Source: CAD feature listing. Evaluate the final solid. Frame: model axes, mm. A direction names the side the tool comes from. Coordinates: 2 decimals unless noted, no trailing zeros. Write each loop counter-clockwise with the first axis right and the second up, starting at its lowest first coordinate (ties: lowest second). Pieces come first, ordered by that corner, then holes. Notation, with made-up numbers: M 78,-4.75 L 124,-4.75 A37 cw 124,31.25 Z; hole C -24,-24 d8. An arc over 180 degrees is marked long. Write item = value, one per line. Start each with the question number.
1. Access query for faces 1 (the face through (14.251, 1.688, -5.637)), 2 (the face through (19.9, 1.7, -25)), 3 (the face through (5, 3, -13)). Directions: +Z, -Z, +X, -X, +Y, -Y. A direction counts if a zero-diameter tool reaches every point of the face in a straight line with its end or side. Return the directions, or none.
2. Line query: line 1 along Z through (x, y) = (2, 16.25); line 2 along X through (y, z) = (5.75, -10.25); line 3 along Z through (x, y) = (14, 3). Output: solid intervals per line, ascending.
3. Section query D-D (y = 7). Output: boundary loops of the cut face in (x, z) (3 decimals), then the cut area to 3 significant figures.
4. Section query A-A (y = 13). Output: boundary loops of the cut face in (x, z), then the cut area to 3 significant figures.
5. Pin query (flat end, axial travel): pin 1 Ø5 at (x, z) = (27.5, -3) entering from +Y; pin 2 Ø1.1 at (x, z) = (37.5, -22.5) entering from +Y; pin 3 Ø5 at (x, z) = (27, -8.5) entering from +Y. Return the tip coordinate at first contact, or that it passes through.
6. Section query B-B (y = 9.5). Output: boundary loops of the cut face in (x, z), then the cut area to 3 significant figures.
7. Pull-direction query (X, two-part tool) for faces 4 (the face through (2.5, 0, -12.3)), 5 (the face through (40, 9, -12)), 6 (the face through (16.479, 1.246, -17.874)); classes: pulls with the +X half, pulls with the -X half, needs draft (parallel to the pull), parting line crosses it, or undercut.
8. Section query C-C (x = 6). Output: boundary loops of the cut face in (y, z), then the cut area to 3 significant figures.
```python
from build123d import *

# Parameters (mm, degrees)
CROQUIS1_W              = 40
CROQUIS1_H              = 25
SALIENTE_EXTRUIR1_DEPTH = 18
CROQUIS2_R              = 16
CORTAR_EXTRUIR1_DEPTH   = 26
CROQUIS3_R              = 1.5
CORTAR_EXTRUIR2_DEPTH   = 19
CORTAR_EXTRUIR3_DEPTH   = 10
SALIENTE_EXTRUIR2_DEPTH = 25
CROQUIS6_W              = 1
CROQUIS6_H              = 25
SALIENTE_EXTRUIR3_DEPTH = 10


with BuildPart() as part:
    # Croquis1 → Saliente-Extruir1 (new body)
    with BuildSketch(Plane(origin=(0, 0, 0), x_dir=(1, 0, 0), z_dir=(0, 1, 0))):
        with Locations((20, 12.5)):
            Rectangle(CROQUIS1_W, CROQUIS1_H)
    extrude(amount=SALIENTE_EXTRUIR1_DEPTH)

    # Croquis2 → Cortar-Extruir1 (cut, through all)
    with BuildSketch(Plane.XY):
        with Locations((20, 18)):
            Circle(CROQUIS2_R)
    extrude(amount=-CORTAR_EXTRUIR1_DEPTH, mode=Mode.SUBTRACT)

    # Croquis3 → Cortar-Extruir2 (cut, through all)
    with BuildSketch(Plane(origin=(0, 18, 0), x_dir=(1, 0, 0), z_dir=(0, 1, 0))):
        with Locations((2, 2.5)):
            Circle(CROQUIS3_R)
        with Locations((2, 22.5)):
            Circle(CROQUIS3_R)
        with Locations((38, 2.5)):
            Circle(CROQUIS3_R)
        with Locations((38, 22.5)):
            Circle(CROQUIS3_R)
    extrude(amount=-CORTAR_EXTRUIR2_DEPTH, mode=Mode.SUBTRACT)

    # Croquis4 → Cortar-Extruir3 (cut)
    with BuildSketch(Plane.XZ):
        with BuildLine():
            Line((12.088237667, -6.478545635), (13.401635398, -5.142871626))
            Line((13.401635398, -5.142871626), (15.124961017, -6.145817155))
            ThreePointArc((15.124961017, -6.145817155), (15.475165724, -6.243431571), (15.828418521, -6.157499195))
            ThreePointArc((15.828418521, -6.157499195), (16.370055517, -5.897538787), (16.933440791, -5.688859407))
            ThreePointArc((16.933440791, -5.688859407), (17.240768872, -5.494639527), (17.414026723, -5.175024714))
            Line((17.414026723, -5.175024714), (17.890921137, -3.238966182))
            Line((17.890921137, -3.238966182), (19.764097728, -3.223214474))
            Line((19.764097728, -3.223214474), (20.273483375, -5.15097929))
            ThreePointArc((20.273483375, -5.15097929), (20.452091683, -5.467635229), (20.762642496, -5.656659312))
            ThreePointArc((20.762642496, -5.656659312), (21.329457457, -5.855834737), (21.875389609, -6.10664968))
            ThreePointArc((21.875389609, -6.10664968), (22.230037574, -6.186629256), (22.578551176, -6.083139256))
            Line((22.578551176, -6.083139256), (24.284766568, -5.051354413))
            Line((24.284766568, -5.051354413), (25.620440577, -6.364752144))
            Line((25.620440577, -6.364752144), (24.617495048, -8.088077763))
            ThreePointArc((24.617495048, -8.088077763), (24.519880632, -8.43828247), (24.605813007, -8.791535267))
            ThreePointArc((24.605813007, -8.791535267), (24.865773416, -9.333172263), (25.074452795, -9.896557537))
            ThreePointArc((25.074452795, -9.896557537), (25.268672676, -10.203885618), (25.588287488, -10.377143469))
            Line((25.588287488, -10.377143469), (27.524346021, -10.854037883))
            Line((27.524346021, -10.854037883), (27.540097728, -12.727214474))
            Line((27.540097728, -12.727214474), (25.612332912, -13.236600121))
            ThreePointArc((25.612332912, -13.236600121), (25.295676973, -13.415208429), (25.106652891, -13.725759242))
            ThreePointArc((25.106652891, -13.725759242), (24.907477465, -14.292574203), (24.656662522, -14.838506355))
            ThreePointArc((24.656662522, -14.838506355), (24.576682946, -15.19315432), (24.680172947, -15.541667922))
            Line((24.680172947, -15.541667922), (25.711957789, -17.247883314))
            Line((25.711957789, -17.247883314), (24.398560059, -18.583557323))
            Line((24.398560059, -18.583557323), (22.67523444, -17.580611794))
            ThreePointArc((22.67523444, -17.580611794), (22.325029732, -17.482997378), (21.971776936, -17.568929753))
            ThreePointArc((21.971776936, -17.568929753), (21.430139939, -17.828890162), (20.866754665, -18.037569541))
            ThreePointArc((20.866754665, -18.037569541), (20.6241928, -18.009408471), (20.386168733, -18.063941468))
            Line((20.386168733, -18.063941468), (19.909274319, -20))
            Line((19.909274319, -20), (18.036097728, -20.015751708))
            Line((18.036097728, -20.015751708), (17.526712081, -18.087986892))
            ThreePointArc((17.526712081, -18.087986892), (17.283728175, -18.036032676), (17.03755296, -18.069769637))
            ThreePointArc((17.03755296, -18.069769637), (16.470737999, -17.870594211), (15.924805848, -17.619779268))
            ThreePointArc((15.924805848, -17.619779268), (15.570157883, -17.539799692), (15.22164428, -17.643289693))
            Line((15.22164428, -17.643289693), (13.515428889, -18.675074535))
            Line((13.515428889, -18.675074535), (12.17975488, -17.361676805))
            Line((12.17975488, -17.361676805), (13.182700409, -15.638351186))
            ThreePointArc((13.182700409, -15.638351186), (13.280314825, -15.288146478), (13.194382449, -14.934893682))
            ThreePointArc((13.194382449, -14.934893682), (13.1083452, -14.769415199), (13.027105933, -14.601529171))
            ThreePointArc((13.027105933, -14.601529171), (13.02605148, -14.489666601), (13.109673231, -14.415358127))
            Line((13.109673231, -14.415358127), (16.284140051, -13.434659859))
            ThreePointArc((16.284140051, -13.434659859), (21.951688309, -11.884896122), (16.306733365, -10.25475669))
            Line((16.306733365, -10.25475669), (13.070699975, -9.410888594))
            ThreePointArc((13.070699975, -9.410888594), (12.983034926, -9.338706443), (12.981392618, -9.2251603))
            ThreePointArc((12.981392618, -9.2251603), (13.060028024, -9.055370844), (13.143532934, -8.887922594))
            ThreePointArc((13.143532934, -8.887922594), (13.22351251, -8.533274629), (13.12002251, -8.184761026))
            Line((13.12002251, -8.184761026), (12.088237667, -6.478545635))
        make_face()
        Polygon((5, -20), (5, -25), (0, -25), (0, -20), (0, -5), (0, 0), (5, 0), (5, -5), align=None)
        Polygon((35, 0), (35, -5), (35, -20), (35, -25), (40, -25), (40, -20), (40, -5), (40, 0), align=None)
    extrude(amount=-CORTAR_EXTRUIR3_DEPTH, mode=Mode.SUBTRACT)

    # Croquis5 → Saliente-Extruir2 (add)
    with BuildSketch(Plane(origin=(0, 0, -25), x_dir=(-1, 0, 0), z_dir=(0, 0, -1))):
        Polygon((-5, 10), (-5, 6), (-3.5, 10), align=None)
        Polygon((-35, 10), (-35, 6), (-36.5, 10), align=None)
    extrude(amount=-SALIENTE_EXTRUIR2_DEPTH)

    # Croquis6 → Saliente-Extruir3 (add)
    with BuildSketch(Plane.XZ.offset(-10)):
        with Locations((0.5, -12.5)):
            Rectangle(CROQUIS6_W, CROQUIS6_H)
        with Locations((39.5, -12.5)):
            Rectangle(CROQUIS6_W, CROQUIS6_H)
        with Locations((2.5, -12.5)):
            Rectangle(CROQUIS6_W, CROQUIS6_H)
        with Locations((37.5, -12.5)):
            Rectangle(CROQUIS6_W, CROQUIS6_H)
    extrude(amount=SALIENTE_EXTRUIR3_DEPTH)


solid = part.part
```
Results are:
q1.face_1 = +Y, -Y
q1.face_2 = -Z, +X, -X, +Y, -Y
q1.face_3 = +Z, -Z, -Y
q2.line_1 = -25 to -24, -21 to -4, -1 to 0
q2.line_2 = 0 to 1, 2 to 3, 5 to 9.71, 30.29 to 35, 37 to 38, 39 to 40
q2.line_3 = -25 to -18.38, -14.14 to -9.65, -5.49 to 0
q3.outline = M 0,-25 L 1,-25 L 1,0 L 0,0 Z; M 2,-25 L 3,-25 L 3,0 L 2,0 Z; M 4.625,-25 L 8.381,-25 L 8.381,0 L 4.625,0 Z; M 31.619,-25 L 35.375,-25 L 35.375,0 L 31.619,0 Z; M 37,-25 L 38,-25 L 38,0 L 37,0 Z; M 39,-25 L 40,-25 L 40,0 L 39,0 Z
q3.area = 288 mm^2
q4.outline = M 0,-25 L 4.8,-25 L 4.8,0 L 0,0 Z; M 35.2,-25 L 40,-25 L 40,0 L 35.2,0 Z; hole C 2,-22.5 d3; hole C 2,-2.5 d3; hole C 38,-22.5 d3; hole C 38,-2.5 d3
q4.area = 212 mm^2
q5.pin_1 = 5.51
q5.pin_2 = 10
q5.pin_3 = 5.13
q6.outline = M 0,-25 L 1,-25 L 1,0 L 0,0 Z; M 2,-25 L 3,-25 L 3,0 L 2,0 Z; M 3.69,-25 L 6.44,-25 L 6.44,0 L 3.69,0 Z; M 33.56,-25 L 36.31,-25 L 36.31,0 L 33.56,0 Z; M 37,-25 L 38,-25 L 38,0 L 37,0 Z; M 39,-25 L 40,-25 L 40,0 L 39,0 Z
q6.area = 238 mm^2
q7.face_4 = needs draft
q7.face_5 = pulls with the +X half
q7.face_6 = undercut
q8.outline = M 0,-25 L 10.25,-25 L 10.25,0 L 0,0 Z
q8.area = 256 mm^2
